from build123d import *

# Parameters (mm, degrees)
F0_W     = 36
F0_H     = 35
F0_R     = 14
F1_DEPTH = 3
F2_R     = 14
F3_DEPTH = 15
F4_R     = 17


with BuildPart() as f1:
    # F0 (on Top) → F1 (new body)
    with BuildSketch(Plane.XY):
        with Locations((0, -17.5)):
            Rectangle(F0_W, F0_H)
        with Locations((0, -17.5)):
            Circle(F0_R, mode=Mode.SUBTRACT)
        with BuildLine():
            Line((-18, 0), (18, 0))
            ThreePointArc((18, 0), (0, 18), (-18, 0))
        make_face()
    extrude(amount=F1_DEPTH)

    # F2 (on face) → F3 (join)
    with BuildSketch(Plane.XY.offset(3)):
        with BuildLine():
            ThreePointArc((15, 0), (0, 15), (-15, 0))
            Line((-15, 0), (15, 0))
        make_face()
        Polygon((-15, 0), (-18, 0), (-18, -35), (18, -35), (18, 0), (15, 0), align=None)
        with Locations((0, -17.5)):
            Circle(F2_R, mode=Mode.SUBTRACT)
    extrude(amount=F3_DEPTH)

    # F4
    f4_edges = [f1.edges().sort_by_distance(p)[0] for p in [
        (-18, -35, 9),
        (18, -35, 9),
    ]]
    fillet(f4_edges, radius=F4_R)


solid = f1.part
The listing builds one solid part. Answer for the finished solid, in the listing's coordinates (mm). A direction names the side the tool comes from. Coordinates: 2 decimals unless noted, no trailing zeros. Write each loop counter-clockwise with the first axis right and the second up, starting at its lowest first coordinate (ties: lowest second). Pieces come first, ordered by that corner, then holes. Notation, with made-up numbers: (21.5, 47) - (54.5, 47) arc R31 cw to (54.5, 85) - close; hole circle Ø11 at (-17, -35.75). An arc over 180 degrees is marked (long way). Answer as CSV lines item,"result".
1. Determine the mould class of faces 4 (the flat face through (17, 0, 10)), 5 (the flat face through (-18, -9, 9)), 6 (the cylindrical face through (-3.03, -31.17, 8.87)) for opening direction X: +X half, -X half, draft (parallel to the pull), parting line (faces both ways), or undercut.
Computed values:
face 4,"draft"
face 5,"-X half"
face 6,"undercut"
2. Find section A-A (x = 0). Give the vertices of the cut face in (y, z), plus the area to 3 significant figures.
Computed values:
outline,"(-35, 0) - (-31.5, 0) - (-31.5, 18) - (-35, 18) - close; (-3.5, 0) - (18, 0) - (18, 3) - (15, 3) - (15, 18) - (-3.5, 18) - close"
area,"405 mm²"
3. Find section B-B (y = -29). Give the vertices of the cut face in (x, z).
Computed values:
outline,"(-13.96, 0) - (-7.98, 0) - (-7.98, 18) - (-13.96, 18) - close; (7.98, 0) - (13.96, 0) - (13.96, 18) - (7.98, 18) - close"
4. Straight lines are drawn through the part: line 1 (Y direction, x = 0, z = 9); line 2 (Y direction, x = 3, z = 6.75); line 3 (X direction, y = -10, z = 2.25). For each, find the intervals that lie inside material, in ascending order. Write a range as [from, to].
Computed values:
line 1,"y = [-35, -31.5], [-3.5, 15]"
line 2,"y = [-34.88, -31.17], [-3.83, 14.7]"
line 3,"x = [-18, -11.82], [11.82, 18]"
5. A tool of negligible diameter and unlimited length cuts with its end or side. For faces 1 (the flat face through (0, 16, 3)), 2 (the flat face through (0, -2, 0)), 3 (the flat face through (-16, 0, 10)), from which of +Z, -Z, +X, -X, +Y, -Y can it reach the whole face along a straight path? Write none if from no direction.
Computed values:
face 1,"+Z, +Y"
face 2,"-Z, +X, -X, +Y, -Y"
face 3,"+Z, -X, +Y"
6. Find section D-D (y = 5). Give the vertices of the cut face in (x, z).
Computed values:
outline,"(-17.29, 0) - (17.29, 0) - (17.29, 3) - (14.14, 3) - (14.14, 18) - (-14.14, 18) - (-14.14, 3) - (-17.29, 3) - close"
7. Find section C-C (z = 15.75). Give the vertices of the cut face in (x, y).
Computed values:
outline,"(-18, -18) arc R17 ccw to (-1, -35) - (1, -35) arc R17 ccw to (18, -18) - (18, 0) - (15, 0) arc R15 ccw to (-15, 0) - (-18, 0) - close; hole circle Ø28 at (0, -17.5)"
8. Given P1, Ø1, axis at x = 3.5, z = 13.5, coming from the +Y side; P2, Ø5, axis at y = -25, z = 8.5, coming from the -X side; P3, Ø2, axis at x = -9.5, z = 6.5, coming from the +Y side; P4, Ø5, axis at x = -4.5, y = -6.5, coming from the +Z side, each flat-ended and moving along its own axis, determine where each tip first touches the part or whether it passes through.
Computed values:
P1,"stops at y = 14.7"
P2,"stops at x = -17.39"
P3,"stops at y = 12.36"
P4,"stops at z = 18"
